```python
from build123d import *

# Parameters (mm, degrees)
SKETCH1_W           = 8
SKETCH1_H           = 10
BOSS_EXTRUDE1_DEPTH = 165
SKETCH2_W           = 8
SKETCH2_H           = 10
BOSS_EXTRUDE2_DEPTH = 22
SKETCH3_W           = 4
SKETCH3_H           = 4
CUT_EXTRUDE1_DEPTH  = 2
SKETCH5_W           = 4
SKETCH5_H           = 4
CUT_EXTRUDE2_DEPTH  = 2


with BuildPart() as part:
    # Sketch1 → Boss-Extrude1 (new body)
    with BuildSketch(Plane.XY):
        with Locations((4, 5)):
            Rectangle(SKETCH1_W, SKETCH1_H)
    extrude(amount=BOSS_EXTRUDE1_DEPTH)

    # Sketch2 → Boss-Extrude2 (add)
    with BuildSketch(Plane(origin=(8, 0, 0), x_dir=(0, 0, -1), z_dir=(1, 0, 0))):
        with Locations((-4, 5)):
            Rectangle(SKETCH2_W, SKETCH2_H)
        with Locations((-161, 5)):
            Rectangle(SKETCH2_W, SKETCH2_H)
    extrude(amount=BOSS_EXTRUDE2_DEPTH)

    # Sketch3 → Cut-Extrude1 (cut)
    with BuildSketch(Plane(origin=(0, 10, 0), x_dir=(1, 0, 0), z_dir=(0, 1, 0))):
        with Locations((4, -82.5)):
            Rectangle(SKETCH3_W, SKETCH3_H)
    extrude(amount=-CUT_EXTRUDE1_DEPTH, mode=Mode.SUBTRACT)

    # Sketch5 → Cut-Extrude2 (cut)
    with BuildSketch(Plane(origin=(8, 0, 0), x_dir=(0, 0, -1), z_dir=(1, 0, 0))):
        with Locations((-82.5, 4)):
            Rectangle(SKETCH5_W, SKETCH5_H)
    extrude(amount=-CUT_EXTRUDE2_DEPTH, mode=Mode.SUBTRACT)


solid = part.part
```
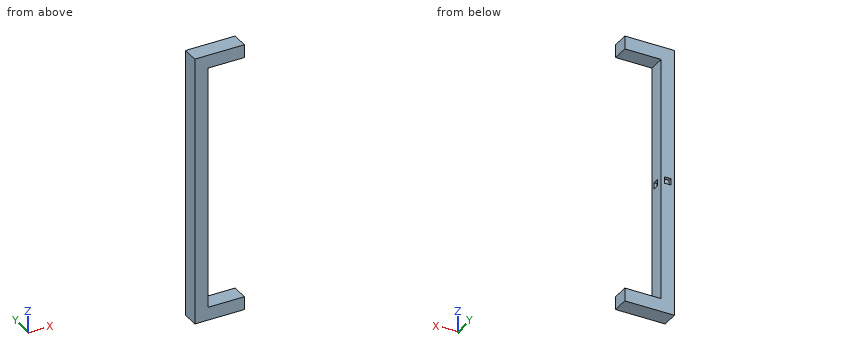
The listing builds one solid part. Answer for the finished solid, in the listing's coordinates (mm). Give positions to 0.01 mm unless a question says otherwise; leave off trailing zeros. Order: outer loops, then holes, each group sorted by start corner. A loop starts at its lowest first (then second) coordinate and runs counter-clockwise, first axis right, second up.
Item 1: The part is cut by section C-C, the plane z = 103. Give the vertices of the cut face in (x, y), and give its area (3 significant figures).
From the geometry:
outline: (0, 0) - (8, 0) - (8, 10) - (0, 10) - close
area: 80.0 mm2
Item 2: Find the intervals of material crossed by probe 1 along Z at (x, y) = (14.75, 5.25); probe 2 along X at (y, z) = (9.5, 17), in increasing order.
From the geometry:
probe 1: z = 0 to 8, 157 to 165
probe 2: x = 0 to 8
Item 3: Given pin 1 Ø5 at (x, z) = (12.5, 38) entering from +Y; pin 2 Ø6 at (y, z) = (3, 140) entering from +X; pin 3 Ø1.2 at (y, z) = (3.5, 83.5) entering from +X, each flat-ended and moving along its own axis, determine where each tip first touches the part or whether it passes through.
From the geometry:
pin 1: passes through
pin 2: stops at x = 8
pin 3: stops at x = 6
Item 4: The part is cut by section B-B, the plane y = 3.75. Give the vertices of the cut face in (x, z), and give its area (3 significant figures).
From the geometry:
outline: (0, 0) - (30, 0) - (30, 8) - (8, 8) - (8, 80.5) - (6, 80.5) - (6, 84.5) - (8, 84.5) - (8, 157) - (30, 157) - (30, 165) - (0, 165) - close
area: 1,660 mm2
Item 5: The part is cut by section A-A, the plane x = 27.5. Give the vertices of the cut face in (y, z), and give its area (3 significant figures).
From the geometry:
outline: (0, 0) - (10, 0) - (10, 8) - (0, 8) - close; (0, 157) - (10, 157) - (10, 165) - (0, 165) - close
area: 160 mm2
